```python
from build123d import *
from OCP.BRepFilletAPI import BRepFilletAPI_MakeChamfer

# Parameters (mm, degrees)
SKETCH1_R           = 13
SKETCH1_R_2         = 10.1
BOSS_EXTRUDE1_DEPTH = 8.5222
CUT_EXTRUDE1_DEPTH  = 21.263955508
CHAMFER1_SIZE       = 1
CHAMFER1_SIZE2      = 0.466307658
FILLET2_R           = 1


with BuildPart() as part:
    # Sketch1 → Boss-Extrude1 (new body)
    with BuildSketch(Plane(origin=(0, 0, 0), x_dir=(1, 0, 0), z_dir=(0, 1, 0))):
        with Locations(Location((0, 0, 0), (0, 0, 270))):
            Circle(SKETCH1_R)
        with Locations(Location((0, 0, 0), (0, 0, 270))):
            Circle(SKETCH1_R_2, mode=Mode.SUBTRACT)
    extrude(amount=BOSS_EXTRUDE1_DEPTH)

    # Sketch2 → Cut-Extrude1 (cut, through all)
    with BuildSketch(Plane.XY):
        with BuildLine():
            Line((-3.175, 4), (-3.175, 0))
            Line((-3.175, 0), (3.175, 0))
            Line((3.175, 0), (3.175, 4))
            ThreePointArc((3.175, 4), (0, 7.175), (-3.175, 4))
        make_face()
    extrude(amount=CUT_EXTRUDE1_DEPTH, mode=Mode.SUBTRACT)

    # Chamfer1: one chamfer whose edges measure the first distance from different faces: ONE call of the kernel's chamfer builder (chamfer() names one face for all edges)
    chamfer1_edges_1 = [part.edges().sort_by_distance(p)[0] for p in [
        (0, 0, -13),
    ]]
    chamfer1_side_1 = [part.faces().sort_by_distance(p)[0] for p in [
        (3.539922426, 0, 11.097151788),
    ]]
    chamfer1_edges_2 = [part.edges().sort_by_distance(p)[0] for p in [
        (0, 8.5222, -13),
    ]]
    chamfer1_side_2 = [part.faces().sort_by_distance(p)[0] for p in [
        (0, 4.2611, -13),
    ]]
    chamfer1_edges_3 = [part.edges().sort_by_distance(p)[0] for p in [
        (0, 0, -10.1),
    ]]
    chamfer1_side_3 = [part.faces().sort_by_distance(p)[0] for p in [
        (0, 4.2611, -10.1),
    ]]
    chamfer1 = BRepFilletAPI_MakeChamfer(part.part.solid().wrapped)
    for e in chamfer1_edges_1:
        chamfer1.Add(CHAMFER1_SIZE, CHAMFER1_SIZE2, e.wrapped, chamfer1_side_1[0].wrapped)  # the first distance lies on this face
    for e in chamfer1_edges_2:
        chamfer1.Add(CHAMFER1_SIZE, CHAMFER1_SIZE2, e.wrapped, chamfer1_side_2[0].wrapped)  # the first distance lies on this face
    for e in chamfer1_edges_3:
        chamfer1.Add(CHAMFER1_SIZE, CHAMFER1_SIZE2, e.wrapped, chamfer1_side_3[0].wrapped)  # the first distance lies on this face
    add(Compound.cast(chamfer1.Shape()), mode=Mode.REPLACE)

    # Fillet2
    fillet2_edges = [part.edges().sort_by_distance(p)[0] for p in [
        (3.175, 0, 10.825180639),
        (-3.175, 0, 10.825180639),
    ]]
    fillet(fillet2_edges, radius=FILLET2_R)


solid = part.part
```
Verification items for the finished model (mm, model axes). A direction names the side the tool comes from. Round coordinates to 2 decimals unless told otherwise and drop trailing zeros. Write each loop counter-clockwise with the first axis right and the second up, starting at its lowest first coordinate (ties: lowest second). Pieces come first, ordered by that corner, then holes. Notation, with made-up numbers: (-39, 79) -> (-4, 79) arc R31 ccw to (-4, 107) -> close; hole circle Ø4 at (-12.5, 51.25). An arc over 180 degrees is marked (long way). Write each question's results on one line, items separated by ' | '.
Q1. Sectioned sample at C-C, the plane y = 5.5. Record the boundary of the cut face in (x, z), and give its area (3 significant figures).
Derived:
outline: (-2.8, 9.7) -> (-2.8, 12.7) arc R13 ccw (long way) to (2.8, 12.7) -> (2.8, 9.7) arc R10.1 cw (long way) to start | area: 194 mm²
Q2. Access from +Z, -Z, +X, -X, +Y, -Y to the whole of each face (thin tool, end or side, straight path). Record for faces 4 (the face through (-7.91, 3.945, -10.316)), 5 (the face through (-3.35, 0.435, 11.118)).
Derived:
face 4: +Y, -Y | face 5: +Z, -Y
Q3. Go/stop test with flat-tipped pins: pin 1 Ø3 at (y, z) = (6, 10) entering from -X; pin 2 Ø4 at (y, z) = (4.5, 7.5) entering from -X; pin 3 Ø3.5 at (y, z) = (3, 11.5) entering from -X. Record where each tip stops, or that it passes through.
Derived:
pin 1: stops at x = -9.84 | pin 2: stops at x = -11.78 | pin 3: stops at x = -8.6
Q4. Sectioned sample at B-B, the plane z = 0. Record the boundary of the cut face in (x, y).
Derived:
outline: (-13, 0.47) -> (-12, 0) -> (-10.57, 0) -> (-10.1, 1) -> (-10.1, 8.52) -> (-12.53, 8.52) -> (-13, 7.52) -> close; (10.1, 1) -> (10.57, 0) -> (12, 0) -> (13, 0.47) -> (13, 7.52) -> (12.53, 8.52) -> (10.1, 8.52) -> close
Q5. Sectioned sample at A-A, the plane x = 0. Record the boundary of the cut face in (y, z) (3 decimals), and give its area (3 significant figures).
Derived:
outline: (0, -12) -> (0.466, -13) -> (7.522, -13) -> (8.522, -12.534) -> (8.522, -10.1) -> (1, -10.1) -> (0, -10.566) -> close; (7.175, 10.1) -> (8.522, 10.1) -> (8.522, 12.534) -> (7.522, 13) -> (7.175, 13) -> close | area: 27.7 mm²
Q6. Draft check along X on faces 1 (the face through (0.5, 0.1, -12.2)), 2 (the face through (0.07, 7.174, 11.27)), 3 (the face through (10.3, 8.522, 0.9)). Enter one of: released by +X, released by -X, zero draft, split by the parting line, or undercut.
Derived:
face 1: split by the parting line | face 2: undercut | face 3: zero draft
Q7. Thickness scan on probe 1 along X at (y, z) = (7, 0); probe 2 along Z at (x, y) = (0, 5); probe 3 along Z at (x, y) = (-0.75, 7.75). Record the ranges inside material, lowest first.
Derived:
probe 1: x = -13 to -10.1, 10.1 to 13 | probe 2: z = -13 to -10.1 | probe 3: z = -12.87 to -10.07, 10.07 to 12.87
